```python
from build123d import *

# Parameters (mm, degrees)
F2_DEPTH = 38.1
F3_R     = 10.6553
F4_DEPTH = 35.56


with BuildPart() as f2:
    # F1 (on Top) → F2 (new body)
    with BuildSketch(Plane.XY):
        with BuildLine():
            Line((-11.1125, -2.921), (-11.1125, 2.232145))
            Line((-11.1125, 2.232145), (-13.265196, 3.886932))
            ThreePointArc((-13.265196, 3.886932), (-14.72113, 4.031284), (-15.494, 2.789007))
            Line((-15.494, 2.789007), (-15.494, -13.912452))
            ThreePointArc((-15.494, -13.912452), (-15.463442, -14.060988), (-15.376731, -14.185399))
            ThreePointArc((-15.376731, -14.185399), (-14.201681, -15.224533), (-12.956605, -16.178644))
            ThreePointArc((-12.956605, -16.178644), (-10.454692, -19.913141), (-11.052133, -24.368373))
            ThreePointArc((-11.052133, -24.368373), (0, -42.896211), (11.052133, -24.368373))
            ThreePointArc((11.052133, -24.368373), (10.454692, -19.913141), (12.956605, -16.178644))
            ThreePointArc((12.956605, -16.178644), (14.201681, -15.224533), (15.376731, -14.185399))
            ThreePointArc((15.376731, -14.185399), (15.463442, -14.060988), (15.494, -13.912452))
            Line((15.494, -13.912452), (15.494, 2.789007))
            ThreePointArc((15.494, 2.789007), (14.72113, 4.031284), (13.265196, 3.886932))
            Line((13.265196, 3.886932), (11.1125, 2.232145))
            Line((11.1125, 2.232145), (11.1125, -2.921))
            Line((11.1125, -2.921), (12.954, -3.518375))
            Line((12.954, -3.518375), (12.954, -12.954))
            ThreePointArc((12.954, -12.954), (6.911881, -16.534312), (0, -17.78))
            ThreePointArc((0, -17.78), (-6.911881, -16.534312), (-12.954, -12.954))
            Line((-12.954, -12.954), (-12.954, -3.518375))
            Line((-12.954, -3.518375), (-11.1125, -2.921))
        make_face()
    extrude(amount=F2_DEPTH)

    # F3 (on face) → F4 (cut)
    with BuildSketch(Plane.XY.offset(38.1)):
        with Locations((0, -30.335911)):
            Circle(F3_R)
    extrude(amount=-F4_DEPTH, mode=Mode.SUBTRACT)


solid = f2.part
```
Source: CAD feature listing. Evaluate the final solid. Frame: model axes, mm. A direction names the side the tool comes from. Round coordinates to 2 decimals unless told otherwise and drop trailing zeros. Loops run counter-clockwise (first coordinate to the right, second up) from the corner with the lowest first, then second, coordinate; pieces in that order, holes last.
1. Section query A-A on y = -10.5. Output: boundary loops of the cut face in (x, z), and give its area (3 significant figures).
2. Contact query for flat-ended pins moving along their axis: pin 1 (17 mm diameter, centred on x = 1, y = -29, fed in from +Z); pin 2 (1 mm diameter, centred on y = -32, z = 30, fed in from -X); pin 3 (6 mm diameter, centred on x = -5.5, z = 5, fed in from +Y). Output: stop coordinate, or through.
3. Section query C-C on x = 9. Output: boundary loops of the cut face in (y, z), and give its area (3 significant figures).
4. Access query for faces 1 (the flat face through (0, -24, 0)), 2 (the flat face through (0, -30, 2.54)), 3 (the flat face through (12.02, -3.216, 18.783)), 4 (the cylindrical face through (-14.22, -15.21, 18.78)), 5 (the flat face through (-11.112, 0, 19)). Directions: +Z, -Z, +X, -X, +Y, -Y. A direction counts if a zero-diameter tool reaches every point of the face in a straight line with its end or side. Return the directions, or none.
5. Ray query, L1, parallel to X at y = -1.5, z = 31; L2, parallel to Y at x = 0.5, z = 11; L3, parallel to X at y = -12, z = 13.5. Return the intervals inside material, ascending.
6. Section query B-B on z = 22. Output: boundary loops of the cut face in (x, y), and give its area (3 significant figures).
7. Section query D-D on y = -28.5. Output: boundary loops of the cut face in (x, z).
8. Mould query, pull axis X, two halves, no side actions, for faces 6 (the flat face through (0, -19, 38.1)), 7 (the flat face through (-12.174, 3.048, 18.783)), 8 (the flat face through (-15.494, -5, 19)). Classes: released by +X, released by -X, zero draft, split by the parting line, or undercut.
Answers below:
1. outline: (-15.49, 0) - (-12.95, 0) - (-12.95, 38.1) - (-15.49, 38.1) - close; (12.95, 0) - (15.49, 0) - (15.49, 38.1) - (12.95, 38.1) - close
1. area: 194 mm2
2. pin 1: stops at z = 2.54
2. pin 2: stops at x = -12.51
2. pin 3: stops at y = -15.86
3. outline: (-39.1, 0) - (-15.62, 0) - (-15.62, 38.1) - (-24.63, 38.1) - (-24.63, 2.54) - (-36.04, 2.54) - (-36.04, 38.1) - (-39.1, 38.1) - close
3. area: 489 mm2
4. face 1: -Z, +X, -X, +Y, -Y
4. face 2: +Z
4. face 3: +Z, -Z
4. face 4: +Z, -Z, -X, -Y
4. face 5: +Z, -Z, +Y
5. L1: x = -15.49 to -11.11, 11.11 to 15.49
5. L2: y = -42.89 to -40.98, -19.69 to -17.77
5. L3: x = -15.49 to -12.95, 12.95 to 15.49
6. outline: (-15.49, -13.91) arc R0.38 ccw to (-15.38, -14.19) arc R22.34 ccw to (-12.96, -16.18) arc R6.35 cw to (-11.05, -24.37) arc R12.56 ccw (long way) to (11.05, -24.37) arc R6.35 cw to (12.96, -16.18) arc R22.34 ccw to (15.38, -14.19) arc R0.38 ccw to (15.49, -13.91) - (15.49, 2.79) arc R1.38 ccw to (13.27, 3.89) - (11.11, 2.23) - (11.11, -2.92) - (12.95, -3.52) - (12.95, -12.95) arc R19.8 cw to (-12.95, -12.95) - (-12.95, -3.52) - (-11.11, -2.92) - (-11.11, 2.23) - (-13.27, 3.89) arc R1.38 ccw to (-15.49, 2.79) - close; hole circle Ø21.31 at (0, -30.34)
6. area: 331 mm2
7. outline: (-12.43, 0) - (12.43, 0) - (12.43, 38.1) - (10.5, 38.1) - (10.5, 2.54) - (-10.5, 2.54) - (-10.5, 38.1) - (-12.43, 38.1) - close
8. face 6: zero draft
8. face 7: undercut
8. face 8: released by -X
